from build123d import *

# Parameters (mm, degrees)
SKETCH1_W          = 2
SKETCH1_H          = 1450
CUT_EXTRUDE1_DEPTH = 1.5
CIRPATTERN1_COUNT  = 4


with BuildPart() as part:
    # Sketch1 → Revolve1 (revolve)
    with BuildSketch(Plane.XY, mode=Mode.PRIVATE) as revolve1_sk:
        with Locations((77.2, 725)):
            Rectangle(SKETCH1_W, SKETCH1_H)
    revolve(revolve1_sk.sketch.rotate(Axis((0, 0, 0), (0, 1, 0)), 90), axis=Axis((0, 0, 0), (0, 1, 0)))

    # Sketch2 → Cut-Extrude1 (cut, symmetric)
    with BuildSketch(Plane.XY):
        Polygon((-185.2, 150), (-185.2, 0), (-78.2, 0), (0, 0), (0, 210), (-78.2, 210), align=None)
    cut_extrude1 = extrude(amount=CUT_EXTRUDE1_DEPTH, both=True, mode=Mode.SUBTRACT)

    # CirPattern1: Cut-Extrude1 ×4 about axis
    cirpattern1_axis = Axis((0, 0, 0), (0, 1, 0))
    for i in range(1, CIRPATTERN1_COUNT):
        add(cut_extrude1.rotate(cirpattern1_axis, i * 360 / CIRPATTERN1_COUNT), mode=Mode.SUBTRACT)


solid = part.part
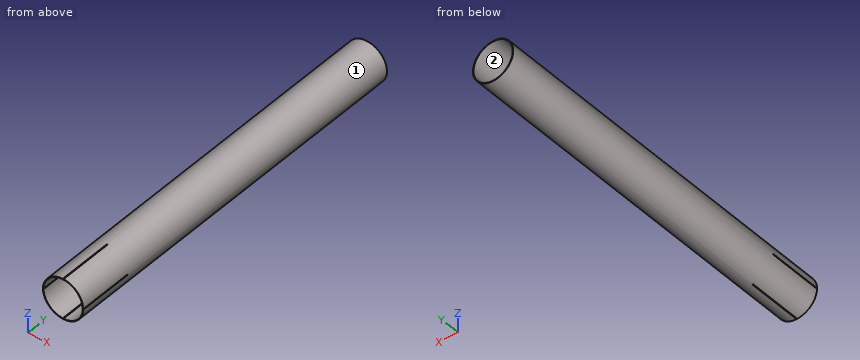
Verification items for the finished model (mm, model axes). Face numbers are marked on the shaded views. Give positions to 0.01 mm unless a question says otherwise; leave off trailing zeros. Loops run counter-clockwise (first coordinate to the right, second up) from the corner with the lowest first, then second, coordinate; pieces in that order, holes last.
1. Cross-section at B-B on z = -63. Record the cut outline in (x, y), and give its area (3 significant figures).
Derived:
outline: (-46.33, 0) - (-42.87, 0) - (-42.87, 1450) - (-46.33, 1450) - close; (42.87, 0) - (46.33, 0) - (46.33, 1450) - (42.87, 1450) - close
area: 10,000 mm2
2. Go/stop test with flat-tipped pins: P1, Ø10, axis at y = 943.5, z = -4, coming from the -X side; P2, Ø1, axis at x = 77, z = 0, coming from the -Y side; P3, Ø6, axis at y = 818, z = -1, coming from the +X side. Record where each tip stops, or that it passes through.
Derived:
P1: stops at x = -78.2
P2: stops at y = 210
P3: stops at x = 78.2
3. Release check for a two-part mould opening along Z. For the marked faces 1 and 2 record: +Z half, -Z half, draft (parallel to the pull), parting line (faces both ways), or undercut.
Derived:
face 1: parting line
face 2: undercut
4. Material ranges on probe 1 along Z at (x, y) = (-6, 170.5); probe 2 along X at (y, z) = (296, 0); probe 3 along X at (y, z) = (1197, 5.5), recorded low to high.
Derived:
probe 1: z = -77.97 to -75.96, 75.96 to 77.97
probe 2: x = -78.2 to -76.2, 76.2 to 78.2
probe 3: x = -78.01 to -76, 76 to 78.01
5. Cross-section at C-C on y = 1098. Record the cut outline in (x, z), and give its area (3 significant figures).
Derived:
outline: circle Ø156.4 at (0, 0); hole circle Ø152.4 at (0, 0)
area: 970 mm2
6. Cross-section at A-A on x = -47.5. Record the cut outline in (y, z), and give its area (3 significant figures).
Derived:
outline: (0, -62.12) - (1450, -62.12) - (1450, -59.58) - (0, -59.58) - close; (0, 59.58) - (1450, 59.58) - (1450, 62.12) - (0, 62.12) - close
area: 7,360 mm2
